from build123d import *

# Parameters (mm, degrees)
F0_W     = 5.08
F0_H     = 304.8
F1_DEPTH = 50.8
F3_DEPTH = 25.4
F5_DEPTH = 101.6
F7_DEPTH = 25.4
F9_DEPTH = 50.8


with BuildPart() as f1:
    # F0 (on Front) → F1 (new body)
    with BuildSketch(Plane.XZ):
        with Locations((-2.54, 13.9935184479)):
            Rectangle(F0_W, F0_H)
    extrude(amount=F1_DEPTH)

    # F2 (on face) → F3 (join)
    with BuildSketch(Plane.XZ.offset(50.8)):
        Polygon((0, 179.0935184479), (0, 166.3935184479), (0, 146.0735184479), (5.08, 146.0735184479), (5.08, 179.0935184479), align=None)
        Polygon((0, 146.0735184479), (0, 166.3935184479), (-5.08, 166.3935184479), (-5.08, -138.4064815521), (0, -138.4064815521), align=None)
    extrude(amount=F3_DEPTH)

    # F4 (on face) → F5 (join)
    with BuildSketch(Plane.XZ.offset(76.2)):
        Polygon((0, 166.3935184479), (-5.08, 166.3935184479), (-5.08, -138.4064815521), (0, -138.4064815521), (0, 146.0735184479), align=None)
    extrude(amount=F5_DEPTH)

    # F6 (on face) → F7 (join)
    with BuildSketch(Plane.XZ.offset(177.8)):
        Polygon((0, 179.0935184479), (0, 166.3935184479), (0, 146.0735184479), (5.08, 146.0735184479), (5.08, 179.0935184479), align=None)
        Polygon((0, 146.0735184479), (0, 166.3935184479), (-5.08, 166.3935184479), (-5.08, -138.4064815521), (0, -138.4064815521), align=None)
    extrude(amount=F7_DEPTH)

    # F8 (on face) → F9 (join)
    with BuildSketch(Plane.XZ.offset(203.2)):
        Polygon((0, 166.3935184479), (-5.08, 166.3935184479), (-5.08, -138.4064815521), (0, -138.4064815521), (0, 146.0735184479), align=None)
    extrude(amount=F9_DEPTH)


solid = f1.part
Design review of the part built by this model. Coordinates are the model's own, in mm. A direction names the side the tool comes from. Coordinates: 2 decimals unless noted, no trailing zeros. Loops run counter-clockwise (first coordinate to the right, second up) from the corner with the lowest first, then second, coordinate; pieces in that order, holes last. Notation, with made-up numbers: (-7, 51) - (19, 51) arc R31 ccw to (19, 75) - close; hole circle Ø9 at (-14, -25). An arc over 180 degrees is marked (long way). Use CSV: the item, a comma, the result in double quotes. Start each with the question number.
1. For faces 1 (the flat face through (-5.08, -125, 16)), 2 (the flat face through (0, -63, 173)), list the 3-axis set-ups (+Z, -Z, +X, -X, +Y, -Y) from which the entire face can be reached by the end or side of a thin tool; tool diameter is ignored.
2. Clearance check with flat-ended pins moving along their axes: pin 1 (2.5 mm diameter, centred on x = 2, z = 169, fed in from -Y); pin 2 (4 mm diameter, centred on y = -65.5, z = 170.5, fed in from -X); pin 3 (2.5 mm diameter, centred on x = 3.5, y = -67.5, fed in from -Z). State where each tip first meets the part, or that it passes through.
3. To check wall thickness, follow probe 1 along Y at (x, z) = (2, 153.5); probe 2 along X at (y, z) = (-78, 50); probe 3 along Z at (x, y) = (2, -183.5). State the ranges of each line that lie inside material, in increasing order.
4. Add section C-C on y = -187.5. Give the boundary of the cut face in (x, z), plus the area to 3 significant figures.
5. Add section D-D on y = -44.5. Give the boundary of the cut face in (x, z).
6. Add section A-A on x = 3.25. Give the boundary of the cut face in (y, z).
7. Add section B-B on z = 152.5. Give the boundary of the cut face in (x, y).
Resolved:
1,face 1,"+Z, -Z, -X, +Y, -Y"
1,face 2,"+Z, -X, +Y, -Y"
2,pin 1,"y = -203.2"
2,pin 2,"x = 0"
2,pin 3,"z = 146.07"
3,probe 1,"-203.2 to -177.8, -76.2 to -50.8"
3,probe 2,"-5.08 to 0"
3,probe 3,"146.07 to 179.09"
4,outline,"(-5.08, -138.41) - (0, -138.41) - (0, 146.07) - (5.08, 146.07) - (5.08, 179.09) - (0, 179.09) - (0, 166.39) - (-5.08, 166.39) - close"
4,area,"1,720 mm2"
5,outline,"(-5.08, -138.41) - (0, -138.41) - (0, 166.39) - (-5.08, 166.39) - close"
6,outline,"(-203.2, 146.07) - (-177.8, 146.07) - (-177.8, 179.09) - (-203.2, 179.09) - close; (-76.2, 146.07) - (-50.8, 146.07) - (-50.8, 179.09) - (-76.2, 179.09) - close"
7,outline,"(-5.08, -254) - (0, -254) - (0, -203.2) - (5.08, -203.2) - (5.08, -177.8) - (0, -177.8) - (0, -76.2) - (5.08, -76.2) - (5.08, -50.8) - (0, -50.8) - (0, 0) - (-5.08, 0) - close"
